Could you check a few things on this model? Use its own coordinates, in mm. A direction names the side the tool comes from. Give positions to 0.01 mm unless a question says otherwise; leave off trailing zeros. Write each loop counter-clockwise with the first axis right and the second up, starting at its lowest first coordinate (ties: lowest second). Pieces come first, ordered by that corner, then holes. Notation, with made-up numbers: M -10.75,57 L -0.75,57 A14 ccw -0.75,61 Z; hole C 80,-8.5 d1. An arc over 180 degrees is marked long. Use one line per item in the form item = value.
Autodesk Inventor part; units mm, degrees
ref_plane "YZ Plane" through (0, 0, 0) normal (1, 0, 0) x (0, 1, 0)
ref_plane "XZ Plane" through (0, 0, 0) normal (0, 1, 0) x (-1, 0, 0)
ref_plane "XY Plane" through (0, 0, 0) normal (0, 0, 1) x (1, 0, 0)
sketch "Skizze1" plane through (0, 0, 0) normal (0, 1, 0) x (-1, 0, 0)
  line L0 (25, 0) -> (-25, 0)
  line L1 (-25, 0) -> (-25, 12)
  line L2 (-25, 12) -> (-8.8574, 101.5958)
  arc A0 (8.8574, 101.5958) -> (-8.8574, 101.5958) centre (0, 100) ccw
  line L3 (8.8574, 101.5958) -> (25, 12)
  line L4 (25, 12) -> (25, 0)
  line L5 (0, 100) -> (0, 0) construction
  dimension "d0" = 100
  dimension "d1" = 12
  dimension "d2" = 50
  dimension "d3" = 9
extrude "Extrusion1" add sketch "Skizze1" along normal blind 3
sketch "Skizze3" plane through (0, 3, 0) normal (0, 1, 0) x (1, 0, 0)
  arc A0 (-8.8574, -101.5958) -> (8.8574, -101.5958) centre (0, -100) ccw
  point P0 (0, 0)
  point P1 (0, -100)
hole "Bohrung1" at (0, 3, 100) direction (0, -1, 0) diameter 10 depth 3
sketch "Skizze4" plane through (0, 3, 0) normal (0, 1, 0) x (1, 0, 0)
  line L0 (-10.7957, -57) -> (10.7957, -57)
  line L1 (10.7957, -57) -> (5.5701, -86.0036)
  arc A0 (-5.5701, -86.0036) -> (5.5701, -86.0036) centre (0, -85) ccw
  line L2 (-5.5701, -86.0036) -> (-10.7957, -57)
  line L3 (25, 0) -> (-25, 0)
  line L4 (8.8574, -101.5958) -> (25, -12)
  line L5 (-25, -12) -> (-8.8574, -101.5958)
  circle A1 centre (0, -100) radius 5
  point P0 (0, 0)
  point P1 (0, 0)
  dimension "d13" = 15
  dimension "d14" = 6
  dimension "d15" = 43
extrude "Extrusion2" cut sketch "Skizze4" against normal up to surface (3 mm away) contours L0 L1 A0 L2
sketch "Skizze5" plane through (0, 3, 0) normal (0, 1, 0) x (1, 0, 0)
  line L0 (13.3181, -43) -> (-13.3181, -43)
  line L1 (-13.3181, -43) -> (-18.543, -14)
  line L2 (-18.543, -14) -> (18.543, -14)
  line L3 (18.543, -14) -> (13.3181, -43)
  line L4 (8.8574, -101.5958) -> (25, -12)
  line L5 (-25, -12) -> (-8.8574, -101.5958)
  line L6 (25, 0) -> (-25, 0)
  line L7 (-10.7957, -57) -> (10.7957, -57)
  point P0 (0, 0)
  point P1 (0, -14)
  point P2 (0, 0)
  dimension "d18" = 6
  dimension "d19" = 14
  dimension "d20" = 14
extrude "Extrusion3" cut sketch "Skizze5" against normal up to surface (3 mm away)
sketch "Skizze6" plane through (0, 3, 0) normal (0, 1, 0) x (1, 0, 0)
  line L0 (25, 0) -> (-25, 0)
  line L1 (-10.7957, -57) -> (10.7957, -57)
  point P0 (0, 0)
  point P1 (0, -50)
  point P2 (0, 0)
  dimension "d30" = 7
hole "Bohrung2" at (0, 3, 50) direction (0, -1, 0) diameter 6 end through all
fillet "Rundung1" radius 2 6 edges at (10.7957, 1.5, 57) (-10.7957, 1.5, 57) (-13.3181, 1.5, 43) (13.3181, 1.5, 43) (18.543, 1.5, 14) (-18.543, 1.5, 14)
sketch "Skizze7" plane through (0, 3, 0) normal (0, 1, 0) x (1, 0, 0)
  line L0 (25, -12) -> (25, 0)
  line L1 (-25, 0) -> (-25, -12)
  line L2 (25, 0) -> (-25, 0)
  point P0 (0, 0)
  point P1 (20, -8)
  point P2 (0, -8)
  point P3 (-20, -8)
  dimension "d39" = 5
  dimension "d40" = 5
  dimension "d41" = 20
  dimension "d42" = 8
hole "Bohrung3" at (20, 3, 8) at (0, 3, 8) at (-20, 3, 8) direction (0, -1, 0) diameter 4 end through all
properties part number "1171" material "Aluminium 6061"
1) Thinking about a two-plate mould opening in X: for faces 3 (the cylindrical face through (0, 1, 47)), 4 (the flat face through (25, 1, 6)), 5 (the cylindrical face through (0, 1, 109)), which applies, released by +X, released by -X, zero draft, split by the parting line, or undercut?
Checked values:
face_3 = undercut
face_4 = released by +X
face_5 = split by the parting line
2) I want a section at B-B, the plane y = 1.4. Please give me the cut outline in (x, z), plus the area to 3 significant figures.
Checked values:
outline = M -25,0 L 25,0 L 25,12 L 8.86,101.6 A9 ccw -8.86,101.6 L -25,12 Z; hole C -20,8 d4; hole M -18.12,16.35 A2 ccw -16.15,14 L 16.15,14 A2 ccw 18.12,16.35 L 13.61,41.35 A2 ccw 11.65,43 L -11.65,43 A2 ccw -13.61,41.35 Z; hole M -10.37,59.35 A2 ccw -8.4,57 L 8.4,57 A2 ccw 10.37,59.35 L 5.57,86 A5.66 ccw -5.57,86 Z; hole C 0,100 d10; hole C 0,50 d6; hole C 0,8 d4; hole C 20,8 d4
area = 2,160 mm2
3) I want a section at C-C, the plane x = 4. Please give me the cut outline in (y, z), plus the area to 3 significant figures.
Checked values:
outline = M 0,0 L 3,0 L 3,14 L 0,14 Z; M 0,43 L 3,43 L 3,57 L 0,57 Z; M 0,89 L 3,89 L 3,97 L 0,97 Z; M 0,103 L 3,103 L 3,108.06 L 0,108.06 Z
area = 123 mm2
4) For pin 1 Ø1.5 at (y, z) = (1.5, 39.5) entering from +X; pin 2 Ø2.5 at (x, z) = (-20, 8) entering from +Y; pin 3 Ø0.9 at (x, y) = (3.5, 1) entering from +Z; pin 4 Ø1.5 at (x, y) = (-1.5, 2.5) entering from +Z, each with a flat end and sliding along its axis, tell me the tip position at first contact or that it passes through.
Checked values:
pin_1 = 20.18
pin_2 = through
pin_3 = 108.47
pin_4 = 108.97
5) For faces 1 (the flat face through (0, 1, 0)), 2 (the flat face through (-15.835, 1.521, 29.03)), which set-ups out of +Z, -Z, +X, -X, +Y, -Y let a thin tool reach every point of the face, with its end or its side?
Checked values:
face_1 = -Z, +X, -X, +Y, -Y
face_2 = +Y, -Y
6) I want a section at D-D, the plane x = 20. Please give me the cut outline in (y, z).
Checked values:
outline = M 0,0 L 3,0 L 3,6 L 0,6 Z; M 0,10 L 3,10 L 3,39.75 L 0,39.75 Z
7) I want a section at A-A, the plane z = 8. Please give me the cut outline in (x, y), plus the area to 3 significant figures.
Checked values:
outline = M -25,0 L -22,0 L -22,3 L -25,3 Z; M -18,0 L -2,0 L -2,3 L -18,3 Z; M 2,0 L 18,0 L 18,3 L 2,3 Z; M 22,0 L 25,0 L 25,3 L 22,3 Z
area = 114 mm2
8) If I drill on L1, parallel to X at y = 2.55, z = 8; L2, parallel to Z at x = 0, y = 1; L3, parallel to Z at x = -4.5, y = 1.7, over which ranges is the centre line in solid material (lowest first)?
Checked values:
L1 = -25 to -22, -18 to -2, 2 to 18, 22 to 25
L2 = 0 to 6, 10 to 14, 43 to 47, 53 to 57, 90.66 to 95, 105 to 109
L3 = 0 to 14, 43 to 57, 88.43 to 97.82, 102.18 to 107.79
